from build123d import *

# Parameters (mm, degrees)
SKETCH1_W           = 16.5
SKETCH1_H           = 16.5
SKETCH1_R           = 1.15
BOSS_EXTRUDE1_DEPTH = 1.6
SKETCH2_W           = 3
SKETCH2_H           = 6.7
BOSS_EXTRUDE2_DEPTH = 2.3
BOSS_EXTRUDE4_DEPTH = 0.3
LPATTERN1_COUNT     = 3
LPATTERN1_PITCH     = 2.54
LPATTERN1_2_COUNT   = 3
LPATTERN1_2_PITCH   = 2.54
SKETCH6_R           = 0.45
CUT_EXTRUDE1_DEPTH  = 18.878216494
FILLET1_R           = 2


with BuildPart() as part:
    # Sketch1 → Boss-Extrude1 (new body)
    with BuildSketch(Plane(origin=(0, 0, 0), x_dir=(1, 0, 0), z_dir=(0, 1, 0))):
        Rectangle(SKETCH1_W, SKETCH1_H)
        with Locations(Location((-5.75, 6, 0), (0, 0, 270))):
            Circle(SKETCH1_R, mode=Mode.SUBTRACT)
        with Locations(Location((5.75, 6, 0), (0, 0, 270))):
            Circle(SKETCH1_R, mode=Mode.SUBTRACT)
    extrude(amount=BOSS_EXTRUDE1_DEPTH)

    # Sketch2 → Boss-Extrude2 (add)
    with BuildSketch(Plane(origin=(0, 1.6, 0), x_dir=(1, 0, 0), z_dir=(0, 1, 0))):
        Rectangle(SKETCH2_W, SKETCH2_H)
    extrude(amount=BOSS_EXTRUDE2_DEPTH)

    # Sketch6 → Cut-Extrude1 (cut, through all)
    with BuildSketch(Plane(origin=(0, 1.6, 0), x_dir=(1, 0, 0), z_dir=(0, 1, 0))):
        with Locations(Location((-5.08, -5.85, 0), (0, 0, 270))):
            Circle(SKETCH6_R)
        with Locations(Location((-2.54, -5.85, 0), (0, 0, 270))):
            Circle(SKETCH6_R)
        with Locations(Location((0, -5.85, 0), (0, 0, 270))):
            Circle(SKETCH6_R)
        with Locations(Location((2.54, -5.85, 0), (0, 0, 270))):
            Circle(SKETCH6_R)
        with Locations(Location((5.08, -5.85, 0), (0, 0, 270))):
            Circle(SKETCH6_R)
    extrude(amount=-CUT_EXTRUDE1_DEPTH, mode=Mode.SUBTRACT)

    # Fillet1
    fillet1_edges = [part.edges().sort_by_distance(p)[0] for p in [
        (8.25, 0.8, 8.25),
        (-8.25, 0.8, 8.25),
        (-8.25, 0.8, -8.25),
        (8.25, 0.8, -8.25),
    ]]
    fillet(fillet1_edges, radius=FILLET1_R)


with BuildPart() as body_2:
    # Sketch4 → Boss-Extrude4 (new, symmetric)
    with BuildSketch(Plane(origin=(0, 0, 0), x_dir=(0, 0, -1), z_dir=(1, 0, 0))):
        with BuildLine():
            Line((-6.15, 0), (-6.15, -0.425))
            ThreePointArc((-6.15, -0.425), (-6.296446609, -0.778553391), (-6.65, -0.925))
            Line((-6.65, -0.925), (-15.55, -0.925))
            Line((-15.55, -0.925), (-15.55, -1.525))
            Line((-15.55, -1.525), (-6.65, -1.525))
            ThreePointArc((-6.65, -1.525), (-5.872182541, -1.202817459), (-5.55, -0.425))
            Line((-5.55, -0.425), (-5.55, 0))
            Line((-5.55, 0), (-6.15, 0))
        make_face()
    extrude(amount=BOSS_EXTRUDE4_DEPTH, both=True)


with BuildPart() as lpattern1_1:
    # LPattern1: pattern copy
    add(body_2.part.moved(Location(Vector(1, 0, 0) * (1 * LPATTERN1_PITCH))))


with BuildPart() as lpattern1_2:
    # LPattern1: pattern copy
    add(body_2.part.moved(Location(Vector(1, 0, 0) * (2 * LPATTERN1_PITCH))))


with BuildPart() as lpattern1_2_1:
    # LPattern1 2: pattern copy
    add(body_2.part.moved(Location(Vector(-1, 0, 0) * (1 * LPATTERN1_2_PITCH))))


with BuildPart() as lpattern1_2_2:
    # LPattern1 2: pattern copy
    add(body_2.part.moved(Location(Vector(-1, 0, 0) * (2 * LPATTERN1_2_PITCH))))


solid = part.part
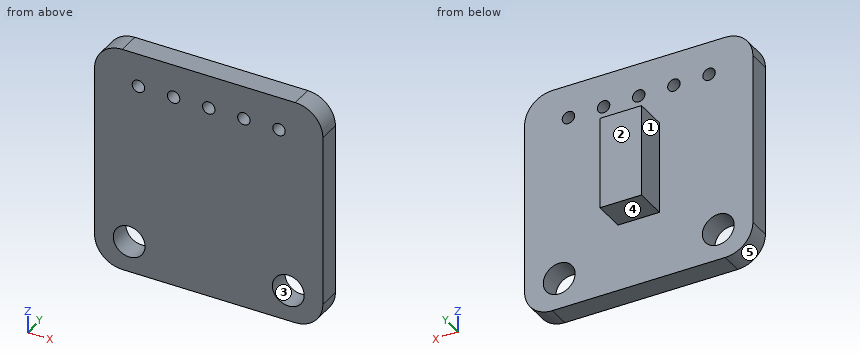
Here's how the part is built. I have some questions about the finished solid (model axes, mm). Face numbers are marked on the shaded views. A direction names the side the tool comes from. Coordinates: 2 decimals unless noted, no trailing zeros. Write each loop counter-clockwise with the first axis right and the second up, starting at its lowest first coordinate (ties: lowest second). Pieces come first, ordered by that corner, then holes. Notation, with made-up numbers: (85.5, 89.5) - (112.5, 89.5) arc R8 cw to (112.5, 95.5) - close; hole circle Ø2 at (66, -40). An arc over 180 degrees is marked (long way). Use one line per item in the form item = value.
1) Suppose I cut it at B-B, the plane z = -6. Write out the boundary of the cut face in (x, y).
Solved:
outline = (-8.25, 0) - (-6.9, 0) - (-6.9, 1.6) - (-8.25, 1.6) - close; (-4.6, 0) - (4.6, 0) - (4.6, 1.6) - (-4.6, 1.6) - close; (6.9, 0) - (8.25, 0) - (8.25, 1.6) - (6.9, 1.6) - close
2) I'm going to push flat-ended pins straight in: P1, Ø0.7, axis at x = 0.5, y = 2, coming from the +Z side; P2, Ø0.7, axis at y = 3, z = -1, coming from the +X side; P3, Ø2.5, axis at x = -5.75, z = -6, coming from the +Y side. Where does each tip first touch, or does it pass through?
Solved:
P1 = 3.35
P2 = 1.5
P3 = 1.6
3) Suppose I cut it at D-D, the plane z = -2.25. Write out the boundary of the cut face in (x, y).
Solved:
outline = (-8.25, 0) - (8.25, 0) - (8.25, 1.6) - (1.5, 1.6) - (1.5, 3.9) - (-1.5, 3.9) - (-1.5, 1.6) - (-8.25, 1.6) - close
4) Suppose I cut it at A-A, the plane x = -2.54. Write out the boundary of the cut face in (y, z), plus the area to 3 significant figures.
Solved:
outline = (0, -8.25) - (1.6, -8.25) - (1.6, 5.4) - (0, 5.4) - close; (0, 6.3) - (1.6, 6.3) - (1.6, 8.25) - (0, 8.25) - close
area = 25.0 mm2
5) On a 3-axis mill with a long thin cutter (end or side, diameter ignored), from which of +Z, -Z, +X, -X, +Y, -Y can I reach the whole of each face in a straight line? I mean the marked faces 4 and 5. Say none if no direction works.
Solved:
face_4 = -Z, +X, -X, +Y
face_5 = -Z, -X, +Y, -Y
6) Thinking about a two-plate mould opening in X: for the marked faces 1, 2 and 3, which applies, released by +X, released by -X, zero draft, split by the parting line, or undercut?
Solved:
face_1 = released by -X
face_2 = zero draft
face_3 = undercut
7) I need wall thicknesses on line 1 (X direction, y = 0.65, z = 5.85); line 2 (X direction, y = 0.4, z = -6); line 3 (Y direction, x = -7.25, z = 0). Which ranges of each line are inside material? Lowest first, please.
Solved:
line_1 = -8.25 to -5.53, -4.63 to -2.99, -2.09 to -0.45, 0.45 to 2.09, 2.99 to 4.63, 5.53 to 8.25
line_2 = -8.25 to -6.9, -4.6 to 4.6, 6.9 to 8.25
line_3 = 0 to 1.6
8) Suppose I cut it at C-C, the plane y = 0.95. Write out the boundary of the cut face in (x, z).
Solved:
outline = (-8.25, -6.25) arc R2 ccw to (-6.25, -8.25) - (6.25, -8.25) arc R2 ccw to (8.25, -6.25) - (8.25, 6.25) arc R2 ccw to (6.25, 8.25) - (-6.25, 8.25) arc R2 ccw to (-8.25, 6.25) - close; hole circle Ø2.3 at (-5.75, -6); hole circle Ø0.9 at (-5.08, 5.85); hole circle Ø0.9 at (-2.54, 5.85); hole circle Ø0.9 at (0, 5.85); hole circle Ø0.9 at (2.54, 5.85); hole circle Ø2.3 at (5.75, -6); hole circle Ø0.9 at (5.08, 5.85)
